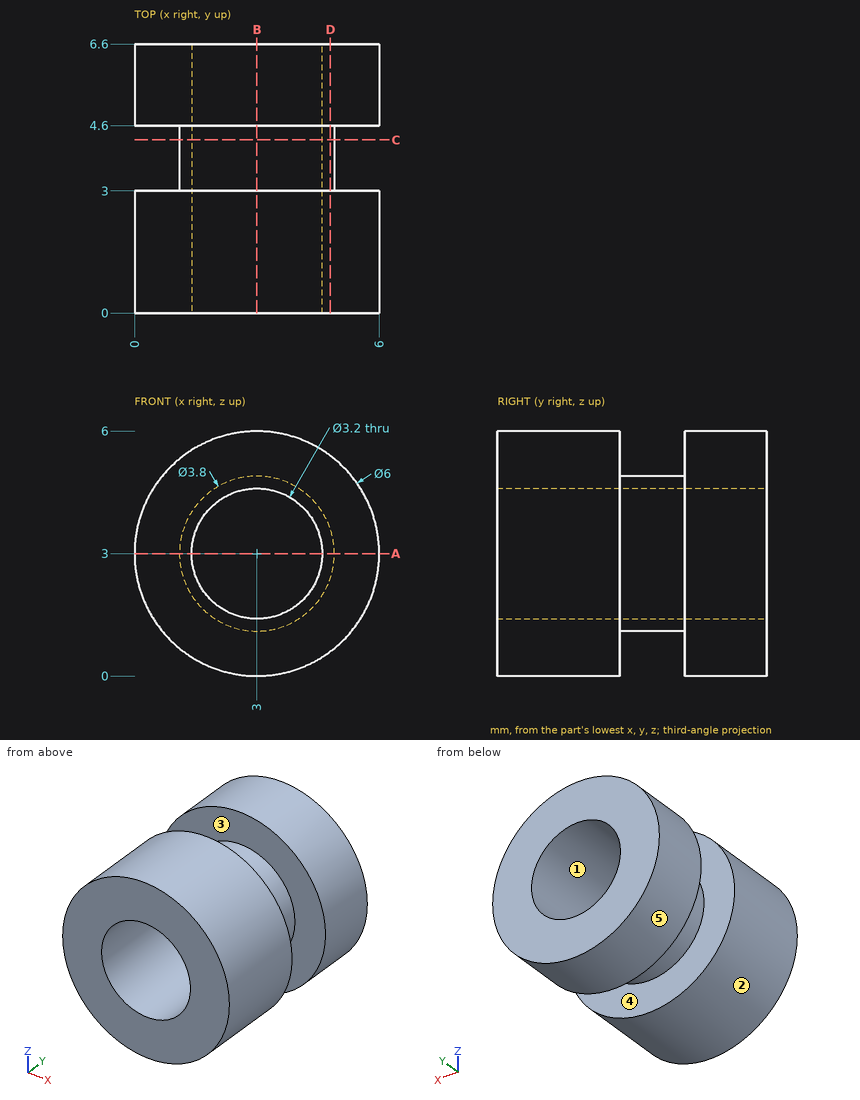
Verification items for this drawing (mm, ordinates from the low corner). A direction names the side the tool comes from. Round coordinates to 2 decimals unless told otherwise and drop trailing zeros. Order: outer loops, then holes, each group sorted by start corner. A loop starts at its lowest first (then second) coordinate and runs counter-clockwise, first axis right, second up. Notation, with made-up numbers: M -36.75,-10 L -19.75,-10 A23 ccw -19.75,1 Z; hole C 57,50 d4. An arc over 180 degrees is marked long. Answer in a Markdown table with one row per item. Add a question column.
Item 1: Material ranges on L1, parallel to Z at x = 3, y = 4.25; L2, parallel to Y at x = 1, z = 1.1; L3, parallel to Z at x = 3, y = 4.75, recorded low to high. Write a range as [from, to].
Item 2: Set-up check for the marked faces 4 and 5: record each of +Z, -Z, +X, -X, +Y, -Y from which the full face is reachable in a straight line by a thin tool's end or side.
Item 3: Depth check by flat-ended pin: pin 1 Ø2 at (y, z) = (5, 1.5) entering from +X. Enter the tip coordinate at first touch or a pass-through.
Item 4: Sectioned sample at B-B, the plane x = 3. Enter the section's corners in (y, z).
Item 5: Draft check along Z on the marked faces 1, 2 and 3. Enter one of: released by +Z, released by -Z, zero draft, split by the parting line, or undercut.
Item 6: Sectioned sample at D-D, the plane x = 4.8. Enter the section's corners in (y, z).
Item 7: Sectioned sample at C-C, the plane y = 4.25. Enter the section's corners in (x, z), plus the area to 3 significant figures.
Item 8: Sectioned sample at A-A, the plane z = 3. Enter the section's corners in (x, y).
Filled in:
| question | item | result |
|---|---|---|
| 1 | L1 | z = [1.1, 1.4], [4.6, 4.9] |
| 1 | L2 | y = [0, 3], [4.6, 6.6] |
| 1 | L3 | z = [0, 1.4], [4.6, 6] |
| 2 | face 4 | none |
| 2 | face 5 | +Y, -Y |
| 3 | pin 1 | stops at x = 5.96 |
| 4 | outline | M 0,0 L 3,0 L 3,1.1 L 4.6,1.1 L 4.6,0 L 6.6,0 L 6.6,1.4 L 0,1.4 Z; M 0,4.6 L 6.6,4.6 L 6.6,6 L 4.6,6 L 4.6,4.9 L 3,4.9 L 3,6 L 0,6 Z |
| 5 | face 1 | undercut |
| 5 | face 2 | split by the parting line |
| 5 | face 3 | zero draft |
| 6 | outline | M 0,0.6 L 3,0.6 L 3,2.39 L 4.6,2.39 L 4.6,0.6 L 6.6,0.6 L 6.6,5.4 L 4.6,5.4 L 4.6,3.61 L 3,3.61 L 3,5.4 L 0,5.4 Z |
| 7 | outline | C 3,3 d3.8; hole C 3,3 d3.2 |
| 7 | area | 3.30 mm² |
| 8 | outline | M 0,0 L 1.4,0 L 1.4,6.6 L 0,6.6 L 0,4.6 L 1.1,4.6 L 1.1,3 L 0,3 Z; M 4.6,0 L 6,0 L 6,3 L 4.9,3 L 4.9,4.6 L 6,4.6 L 6,6.6 L 4.6,6.6 Z |
